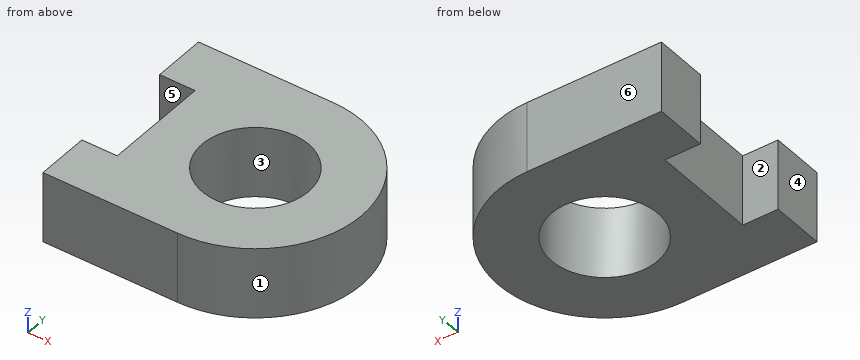
from build123d import *

# Parameters (mm, degrees)
F0_R     = 15
F1_DEPTH = 10


with BuildPart() as f1:
    # F0 (on Top) → F1 (new body, symmetric)
    with BuildSketch(Plane.XY):
        with BuildLine():
            Line((-38, -30), (0, -30))
            ThreePointArc((0, -30), (30, 0), (0, 30))
            Line((0, 30), (-38, 30))
            Line((-38, 30), (-38, 15))
            Line((-38, 15), (-28, 15))
            Line((-28, 15), (-28, -15))
            Line((-28, -15), (-38, -15))
            Line((-38, -15), (-38, -30))
        make_face()
        Circle(F0_R, mode=Mode.SUBTRACT)
    extrude(amount=F1_DEPTH, both=True)


solid = f1.part
Can you work these out from the model? Positions are in its coordinate system, mm. Face numbers are marked on the shaded views. A direction names the side the tool comes from. Give positions to 0.01 mm unless a question says otherwise; leave off trailing zeros. Write each loop counter-clockwise with the first axis right and the second up, starting at its lowest first coordinate (ties: lowest second). Pieces come first, ordered by that corner, then holes. Notation, with made-up numbers: M 0.5,-36.5 L 20.5,-36.5 A15 cw 20.5,-15.5 Z; hole C 38.25,9.5 d6. An arc over 180 degrees is marked long. Answer in a Markdown table with one row per item. Add a question column.
Item 1: Please list where these lines run through material, in increasing order: L1, parallel to Y at x = -5, z = -6.5; L2, parallel to Y at x = -10, z = 6; L3, parallel to X at y = -11, z = -6.25.
Item 2: On a 3-axis mill with a long thin cutter (end or side, diameter ignored), from which of +Z, -Z, +X, -X, +Y, -Y can I reach the whole of each face in a straight line? I mean the marked faces 5 and 6. Say none if no direction works.
Item 3: Imagine slicing it at D-D, the plane x = 20. Write out the boundary of the cut face in (y, z).
Item 4: For pin 1 Ø12 at (x, y) = (-31, 12.5) entering from +Z; pin 2 Ø5 at (y, z) = (-10, 3.5) entering from +X; pin 3 Ø1 at (y, z) = (11.5, 8) entering from -X; pin 4 Ø4 at (x, y) = (-30.5, 6.5) entering from +Z, each with a flat end and sliding along its axis, tell me the tip position at first contact or that it passes through.
Item 5: Imagine slicing it at A-A, the plane y = 0. Write out the boundary of the cut face in (x, z), plus the area to 3 significant figures.
Item 6: Imagine slicing it at C-C, the plane x = -13. Write out the boundary of the cut face in (y, z), plus the area to 3 significant figures.
Item 7: We'd pull the mould along X, two halves only. Please class the marked faces 1, 2, 3 and 4: released by +X, released by -X, zero draft, split by the parting line, or undercut.
Item 8: Imagine slicing it at B-B, the plane z = -6. Write out the boundary of the cut face in (x, y), plus the area to 3 significant figures.
Evaluation:
| question | item | result |
|---|---|---|
| 1 | L1 | y = -30 to -14.14, 14.14 to 30 |
| 1 | L2 | y = -30 to -11.18, 11.18 to 30 |
| 1 | L3 | x = -28 to -10.2, 10.2 to 27.91 |
| 2 | face 5 | +Z, -Z, -X |
| 2 | face 6 | +Z, -Z, +X, -X, +Y |
| 3 | outline | M -22.36,-10 L 22.36,-10 L 22.36,10 L -22.36,10 Z |
| 4 | pin 1 | stops at z = 10 |
| 4 | pin 2 | stops at x = 29.05 |
| 4 | pin 3 | stops at x = -28 |
| 4 | pin 4 | passes through |
| 5 | outline | M -28,-10 L -15,-10 L -15,10 L -28,10 Z; M 15,-10 L 30,-10 L 30,10 L 15,10 Z |
| 5 | area | 560 mm² |
| 6 | outline | M -30,-10 L -7.48,-10 L -7.48,10 L -30,10 Z; M 7.48,-10 L 30,-10 L 30,10 L 7.48,10 Z |
| 6 | area | 901 mm² |
| 7 | face 1 | released by +X |
| 7 | face 2 | zero draft |
| 7 | face 3 | undercut |
| 7 | face 4 | released by -X |
| 8 | outline | M -38,-30 L 0,-30 A30 ccw 0,30 L -38,30 L -38,15 L -28,15 L -28,-15 L -38,-15 Z; hole C 0,0 d30 |
| 8 | area | 2,690 mm² |
